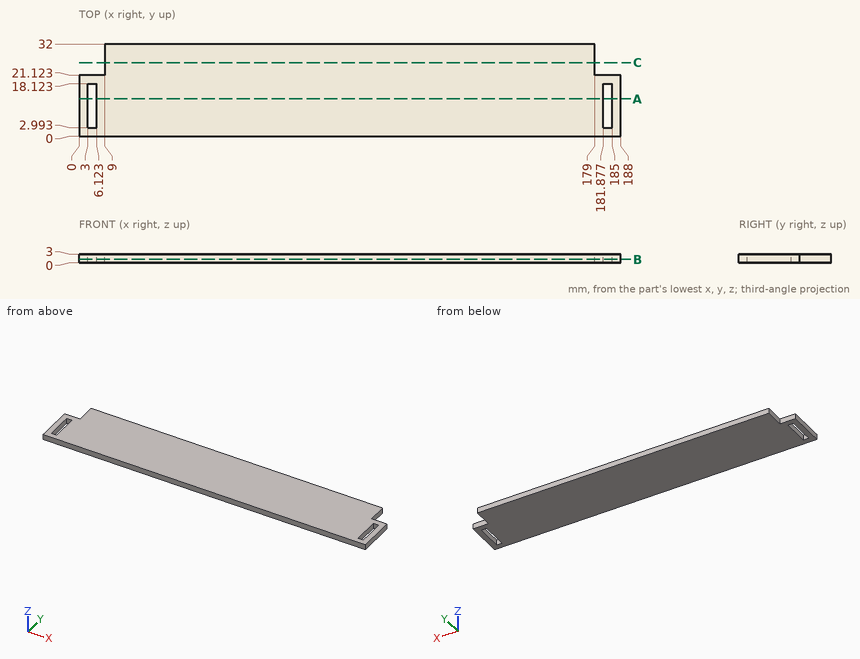
Check sheet for the drawn part. Datum: minimum x, y, z corner. Units: mm. Coordinates: 2 decimals unless noted, no trailing zeros. Order: outer loops, then holes, each group sorted by start corner. A loop starts at its lowest first (then second) coordinate and runs counter-clockwise, first axis right, second up. Notation, with made-up numbers: (-39, -36.75) -> (-14, -36.75) arc R30 ccw to (-14, 2.25) -> close; hole circle Ø7 at (2.5, 28.5). An arc over 180 degrees is marked (long way). Write each question's results on one line, items separated by ' | '. Start each with the question number.
1) Section check C-C (y = 25.5). Enter the section's corners in (x, z).
2) Material ranges on line 1 along X through (y, z) = (9, 2.5); line 2 along X through (y, z) = (25, 0.95), recorded low to high.
3) Section check A-A (y = 13). Enter the section's corners in (x, z), and give its area (3 significant figures).
4) Depth check by flat-ended pin: pin 1 (12 mm diameter, centred on x = 62.5, y = 27.5, fed in from -Z); pin 2 (1.5 mm diameter, centred on x = 3, z = 1, fed in from +Y). Enter the tip coordinate at first touch or a pass-through.
5) Section check B-B (z = 1.25). Enter the section's corners in (x, y), and give its area (3 significant figures).
Checked values:
1) outline: (9, 0) -> (179, 0) -> (179, 3) -> (9, 3) -> close
2) line 1: 0 to 3, 6.12 to 181.88, 185 to 188 | line 2: 9 to 179
3) outline: (0, 0) -> (3, 0) -> (3, 3) -> (0, 3) -> close; (6.12, 0) -> (181.88, 0) -> (181.88, 3) -> (6.12, 3) -> close; (185, 0) -> (188, 0) -> (188, 3) -> (185, 3) -> close | area: 545 mm²
4) pin 1: z = 0 | pin 2: y = 21.12
5) outline: (0, 0) -> (188, 0) -> (188, 21.12) -> (179, 21.12) -> (179, 32) -> (9, 32) -> (9, 21.12) -> (0, 21.12) -> close; hole (3, 2.99) -> (6.12, 2.99) -> (6.12, 18.12) -> (3, 18.12) -> close; hole (181.88, 2.99) -> (185, 2.99) -> (185, 18.12) -> (181.88, 18.12) -> close | area: 5,730 mm²
